```python
from build123d import *

# Parameters (mm, degrees)
SKETCH1_W           = 50
SKETCH1_H           = 70
BOSS_EXTRUDE1_DEPTH = 100
CUT_EXTRUDE1_DEPTH  = 100


with BuildPart() as part:
    # Sketch1 → Boss-Extrude1 (new body)
    with BuildSketch(Plane(origin=(0, 0, 0), x_dir=(0, 0, -1), z_dir=(1, 0, 0))):
        with Locations((25, 35)):
            Rectangle(SKETCH1_W, SKETCH1_H)
    extrude(amount=BOSS_EXTRUDE1_DEPTH)

    # Sketch2 → Cut-Extrude1 (cut)
    with BuildSketch(Plane(origin=(100, 0, 0), x_dir=(0, 0, -1), z_dir=(1, 0, 0))):
        Polygon((0, 70), (30, 70), (10, 20), (0, 20), align=None)
    extrude(amount=-CUT_EXTRUDE1_DEPTH, mode=Mode.SUBTRACT)

    # Mirror1: part across plane


with BuildPart() as part_1:
    add(part.part)
    add(part.part.mirror(Plane.XY))


solid = part_1.part
```
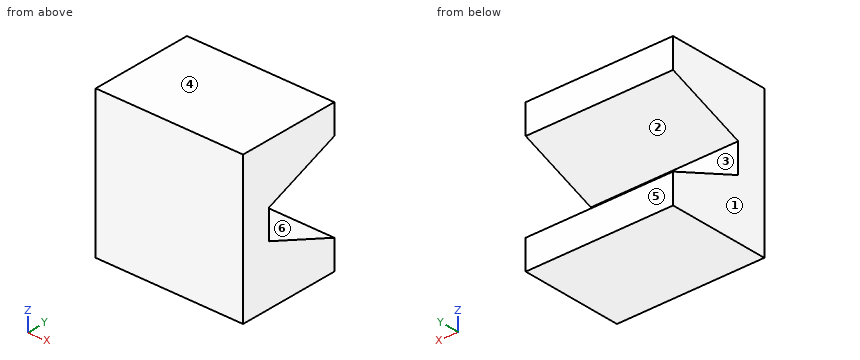
Verification items for the finished model (mm, model axes). Face numbers are marked on the shaded views. A direction names the side the tool comes from. Coordinates: 2 decimals unless noted, no trailing zeros. Write each loop counter-clockwise with the first axis right and the second up, starting at its lowest first coordinate (ties: lowest second). Pieces come first, ordered by that corner, then holes. Notation, with made-up numbers: (42, -39.5) - (97, -39.5) arc R17 ccw to (97, -28.5) - close; hole circle Ø5 at (48.5, -27.75). An arc over 180 degrees is marked (long way). Write item = value, one per line.
Q1. Cross-section at C-C (x = 19). Enter the section's corners in (y, z).
Answer:
outline = (0, -50) - (70, -50) - (70, -30) - (20, -10) - (20, 10) - (70, 30) - (70, 50) - (0, 50) - close
Q2. Cross-section at D-D (z = 5). Enter the section's corners in (x, y), plus the area to 3 significant figures.
Answer:
outline = (0, 0) - (100, 0) - (100, 20) - (0, 20) - close
area = 2,000 mm²
Q3. Go/stop test with flat-tipped pins: pin 1 Ø6 at (x, z) = (37.5, 3) entering from +Y; pin 2 Ø3 at (x, z) = (58.5, -12.5) entering from +Y. Record where each tip stops, or that it passes through.
Answer:
pin_1 = 20
pin_2 = 30
Q4. Mould release check, pull along Z, two halves, no side actions. Record for the marked faces 3, 4, 5 and 6: released by +Z, released by -Z, zero draft, split by the parting line, or undercut.
Answer:
face_3 = undercut
face_4 = released by +Z
face_5 = zero draft
face_6 = undercut
Q5. Material ranges on L1, parallel to Y at x = 63, z = -1; L2, parallel to Z at x = 91, y = 63; L3, parallel to Z at x = 20, y = 52, recorded low to high. Write a range as from..to.
Answer:
L1 = 0..20
L2 = -50..-27.2, 27.2..50
L3 = -50..-22.8, 22.8..50
Q6. Cross-section at B-B (y = 56). Enter the section's corners in (x, z).
Answer:
outline = (0, -50) - (100, -50) - (100, -24.4) - (0, -24.4) - close; (0, 24.4) - (100, 24.4) - (100, 50) - (0, 50) - close
Q7. Access from +Z, -Z, +X, -X, +Y, -Y to the whole of each face (thin tool, end or side, straight path). Record for the marked faces 1 and 2.
Answer:
face_1 = +Z, -Z, -X, +Y, -Y
face_2 = +X, -X, +Y
Q8. Cross-section at A-A (y = 46.5). Enter the section's corners in (x, z), plus the area to 3 significant figures.
Answer:
outline = (0, -50) - (100, -50) - (100, -20.6) - (0, -20.6) - close; (0, 20.6) - (100, 20.6) - (100, 50) - (0, 50) - close
area = 5,880 mm²
